from build123d import *

# Parameters (mm, degrees)
SKETCH2_W              = 38.1
SKETCH2_H              = 25.4
BOSS_EXTRUDE1_DEPTH    = 3.175
SKETCH20_W             = 46.99
SKETCH20_H             = 25.4
BOSS_EXTRUDE5_DEPTH    = 3.175
SKETCH25_W             = 43.815
SKETCH25_H             = 25.4
BOSS_EXTRUDE6_DEPTH    = 3.175
CONVERT_SOLID2_START   = -12.7
CONVERT_SOLID2_DEPTH   = 25.4
CONVERT_SOLID2_2_DEPTH = 25.4
SKETCH16_W             = 25.4
SKETCH16_H             = 88.9
BOSS_EXTRUDE3_DEPTH    = 3.175
SKETCH17_R             = 3.175
CUT_EXTRUDE1_DEPTH     = 114.549648172
FILLET1_R              = 2.54


# Read off the part's stored shape, not the designer's step: Convert-Solid2
with BuildPart() as part:
    # Sketch2 → Boss-Extrude1 (new body)
    with BuildSketch(Plane.XY):
        Rectangle(SKETCH2_W, SKETCH2_H)
    extrude(amount=BOSS_EXTRUDE1_DEPTH)

    # Sketch20 → Boss-Extrude5 (add)
    with BuildSketch(Plane.ZY.offset(19.05)):
        with Locations((23.495, 0)):
            Rectangle(SKETCH20_W, SKETCH20_H)
    extrude(amount=-BOSS_EXTRUDE5_DEPTH)

    # Sketch25 → Boss-Extrude6 (add)
    with BuildSketch(Plane(origin=(19.05, 0, 0), x_dir=(0, 0, -1), z_dir=(1, 0, 0))):
        with Locations((-21.9075, 0)):
            Rectangle(SKETCH25_W, SKETCH25_H)
    extrude(amount=-BOSS_EXTRUDE6_DEPTH)

    # Convert-Solid2 outline → Convert-Solid2 (cut)
    with BuildSketch(Plane(origin=(0, 0, 0), x_dir=(1, 0, 0), z_dir=(0, 1, 0)).offset(CONVERT_SOLID2_START)):
        with BuildLine():
            Line((19.05, 0), (12.7, 0))
            ThreePointArc((12.7, 0), (17.190128061, -1.859871939), (19.05, -6.35))
            Line((19.05, -6.35), (19.05, 0))
        make_face()
        with BuildLine():
            ThreePointArc((-19.05, -6.35), (-17.190128061, -1.859871939), (-12.7, 0))
            Line((-12.7, 0), (-19.05, 0))
            Line((-19.05, 0), (-19.05, -6.35))
        make_face()
    extrude(amount=CONVERT_SOLID2_DEPTH, mode=Mode.SUBTRACT)

    # Convert-Solid2 2 outline → Convert-Solid2 2 (add)
    with BuildSketch(Plane(origin=(0, 0, 0), x_dir=(1, 0, 0), z_dir=(0, 1, 0)).offset(CONVERT_SOLID2_START)):
        with BuildLine():
            Line((15.875, -3.175), (12.7, -3.175))
            ThreePointArc((12.7, -3.175), (14.94506403, -4.10493597), (15.875, -6.35))
            Line((15.875, -6.35), (15.875, -3.175))
        make_face()
        with BuildLine():
            ThreePointArc((-15.875, -6.35), (-14.94506403, -4.10493597), (-12.7, -3.175))
            Line((-12.7, -3.175), (-15.875, -3.175))
            Line((-15.875, -3.175), (-15.875, -6.35))
        make_face()
    extrude(amount=CONVERT_SOLID2_2_DEPTH)

    # Sketch16 → Boss-Extrude3 (add)
    with BuildSketch(Plane(origin=(0, 0, 0), x_dir=(-1, 0, 0), z_dir=(0, 0, -1))):
        with Locations((0, 57.15)):
            Rectangle(SKETCH16_W, SKETCH16_H)
    extrude(amount=-BOSS_EXTRUDE3_DEPTH)

    # Sketch17 → Cut-Extrude1 (cut, through all)
    with BuildSketch(Plane(origin=(0, 0, 0), x_dir=(-1, 0, 0), z_dir=(0, 0, -1))):
        with Locations((0, 88.9)):
            Circle(SKETCH17_R)
    extrude(amount=-CUT_EXTRUDE1_DEPTH, mode=Mode.SUBTRACT)

    # Fillet1
    fillet1_edges = [part.edges().sort_by_distance(p)[0] for p in [
        (12.7, 101.6, 1.5875),
        (-12.7, 101.6, 1.5875),
    ]]
    fillet(fillet1_edges, radius=FILLET1_R)


solid = part.part
Input: part model. Units: mm. Frame: model coordinates. A direction names the side the tool comes from. Round coordinates to 2 decimals unless told otherwise and drop trailing zeros. Loops run counter-clockwise (first coordinate to the right, second up) from the corner with the lowest first, then second, coordinate; pieces in that order, holes last. Notation, with made-up numbers: (6.5, 37) -> (17.5, 37) arc R19 ccw to (17.5, 41) -> close; hole circle Ø1 at (-26.5, 19). An arc over 180 degrees is marked (long way). Answer as a JSON object with one key per item and string values. Group by question number.
1) Section query B-B on x = 0. Output: boundary loops of the cut face in (y, z) (3 decimals), plus the area to 3 significant figures.
2) Ray query, L1, parallel to Y at x = 0, z = 2.1 (3 decimals); L2, parallel to X at y = 11, z = 15.5 (3 decimals); L3, parallel to Z at x = -12, y = 36.5 (3 decimals). Return the intervals inside material, ascending.
3) Pin query (flat end, axial travel): pin 1 (2.5 mm diameter, centred on y = 54, z = 2.5, fed in from -X); pin 2 (12.5 mm diameter, centred on x = 0.5, y = 36, fed in from +Z) (3 decimals); pin 3 (3 mm diameter, centred on x = 16.5, z = 20.5, fed in from +Y). Return the tip coordinate at first contact, or that it passes through.
4) Draft query along X for faces 1 (the cylindrical face through (14.92, -0.18, 4.08)), 2 (the flat face through (-12.7, 55, 2)), 3 (the flat face through (17, 0, 43.815)). Return one class per face: +X half, -X half, draft (parallel to the pull), parting line (faces both ways), or undercut.
5) Section query A-A on z = 31.5. Output: boundary loops of the cut face in (x, y) (3 decimals), plus the area to 3 significant figures.
6) Reachability of faces 4 (the flat face through (15.875, 0, 25)), 5 (the flat face through (-17, 12.7, 23)), 6 (the flat face through (12.7, 55, 2)), 7 (the flat face through (0, 101.6, 2)) from +Z, -Z, +X, -X, +Y, -Y: full face, straight path, thin tool, end or side. Return the list, or none.
7) Section query C-C on y = 8. Output: boundary loops of the cut face in (x, z) (3 decimals), plus the area to 3 significant figures.
8) Section query D-D on y = 71. Output: boundary loops of the cut face in (x, z) (3 decimals).
Reply:
{
 "1": {"outline": "(-12.7, 0) -> (85.725, 0) -> (85.725, 3.175) -> (-12.7, 3.175) -> close; (92.075, 0) -> (101.6, 0) -> (101.6, 3.175) -> (92.075, 3.175) -> close", "area": "343 mm2"},
 "2": {"L1": "y = -12.7 to 85.725, 92.075 to 101.6", "L2": "x = -19.05 to -15.875, 15.875 to 19.05", "L3": "z = 0 to 3.175"},
 "3": {"pin 1": "stops at x = -12.7", "pin 2": "stops at z = 3.175", "pin 3": "stops at y = 12.7"},
 "4": {"face 1": "undercut", "face 2": "-X half", "face 3": "draft"},
 "5": {"outline": "(-19.05, -12.7) -> (-15.875, -12.7) -> (-15.875, 12.7) -> (-19.05, 12.7) -> close; (15.875, -12.7) -> (19.05, -12.7) -> (19.05, 12.7) -> (15.875, 12.7) -> close", "area": "161 mm2"},
 "6": {"face 4": "+Z, +Y, -Y", "face 5": "+Z, -Z, -X, +Y", "face 6": "+Z, -Z, +X, +Y", "face 7": "+Z, -Z, +X, -X, +Y"},
 "7": {"outline": "(-19.05, 6.35) arc R6.35 ccw to (-12.7, 0) -> (12.7, 0) arc R6.35 ccw to (19.05, 6.35) -> (19.05, 43.815) -> (15.875, 43.815) -> (15.875, 6.35) arc R3.175 cw to (12.7, 3.175) -> (-12.7, 3.175) arc R3.175 cw to (-15.875, 6.35) -> (-15.875, 46.99) -> (-19.05, 46.99) -> close", "area": "376 mm2"},
 "8": {"outline": "(-12.7, 0) -> (12.7, 0) -> (12.7, 3.175) -> (-12.7, 3.175) -> close"}
}
